Geometry check sheet. Reference: the model listing, model coordinates, mm. A direction names the side the tool comes from. Give positions to 0.01 mm unless a question says otherwise; leave off trailing zeros. Loops run counter-clockwise (first coordinate to the right, second up) from the corner with the lowest first, then second, coordinate; pieces in that order, holes last. Notation, with made-up numbers: (54.25, 50.25) -> (67.25, 50.25) arc R22 ccw to (67.25, 83.25) -> close; hole circle Ø1 at (-20, 51.5). An arc over 180 degrees is marked (long way). Answer in a Markdown table with one row per item. Add a question column.
```python
from build123d import *

# Parameters (mm, degrees)
SZKIC1_W                    = 70
SZKIC1_H                    = 100
DODANIE_WYCI_GNI_CIE1_DEPTH = 10
SZKIC2_R                    = 10
DODANIE_WYCI_GNI_CIE2_DEPTH = 30
SZKIC3_R                    = 15
DODANIE_WYCI_GNI_CIE3_DEPTH = 60
WYTNIJ_WYCI_GNI_CIE1_DEPTH  = 30


with BuildPart() as part:
    # Szkic1 → Dodanie-wyciągnięcie1 (new body)
    with BuildSketch(Plane.XY):
        Rectangle(SZKIC1_W, SZKIC1_H)
    extrude(amount=DODANIE_WYCI_GNI_CIE1_DEPTH)

    # Szkic2 → Dodanie-wyciągnięcie2 (add)
    with BuildSketch(Plane(origin=(0, 0, 0), x_dir=(-1, 0, 0), z_dir=(0, 0, -1))):
        Circle(SZKIC2_R)
    extrude(amount=DODANIE_WYCI_GNI_CIE2_DEPTH)

    # Szkic3 → Dodanie-wyciągnięcie3 (add)
    with BuildSketch(Plane(origin=(0, 0, -30), x_dir=(-1, 0, 0), z_dir=(0, 0, -1))):
        Circle(SZKIC3_R)
    extrude(amount=DODANIE_WYCI_GNI_CIE3_DEPTH)

    # Szkic4 → Wytnij-wyciągnięcie1 (cut, symmetric)
    with BuildSketch(Plane(origin=(0, 0, 0), x_dir=(0, 0, -1), z_dir=(1, 0, 0))):
        Polygon((83.125666523, 15), (44.759974282, -15), (90, -15), (90, 15), align=None)
    extrude(amount=WYTNIJ_WYCI_GNI_CIE1_DEPTH, both=True, mode=Mode.SUBTRACT)


solid = part.part
```
1. Sectioned sample at C-C (y = -13). Enter the section's corners in (x, z).
2. Gauge pin test, flat ends, axial feed: pin 1 Ø1.5 at (x, z) = (1, -35) entering from -Y; pin 2 Ø6 at (x, z) = (-19.5, -55) entering from +Y; pin 3 Ø10 at (x, y) = (-26, -1) entering from -Z; pin 4 Ø12 at (x, z) = (-16.5, -52.5) entering from +Y. Record the tip position at first contact, or that the pin passes through.
3. Sectioned sample at A-A (x = -11.5). Enter the section's corners in (y, z).
4. Access from +Z, -Z, +X, -X, +Y, -Y to the whole of each face (thin tool, end or side, straight path). Record for faces 5 (the face through (1.953, 14.872, -50.288)), 6 (the face through (0, -50, 5)).
5. Sectioned sample at B-B (x = 0). Enter the section's corners in (y, z).
6. Release check for a two-part mould opening along Z. For faces 1 (the face through (2.17, -9.76, -14.79)), 2 (the face through (0, 50, 5)), 3 (the face through (0.2, 0.2, -64.2)), 4 (the face through (-3, -10, -30)) record: released by +Z, released by -Z, zero draft, split by the parting line, or undercut.
7. Sectioned sample at D-D (z = -40). Enter the section's corners in (x, y), plus the area to 3 significant figures.
8. Material ranges on L1, parallel to Z at x = 13.5, y = -18; L2, parallel to Z at x = 8.5, y = 6; L3, parallel to X at y = 2.5, z = -40, recorded low to high. Write a range as from..to.
Response:
| question | item | result |
|---|---|---|
| 1 | outline | (-35, 0) -> (35, 0) -> (35, 10) -> (-35, 10) -> close; (-7.48, -47.32) -> (7.48, -47.32) -> (7.48, -30) -> (-7.48, -30) -> close |
| 2 | pin 1 | stops at y = -15 |
| 2 | pin 2 | passes through |
| 2 | pin 3 | stops at z = 0 |
| 2 | pin 4 | stops at y = 10.71 |
| 3 | outline | (-50, 0) -> (50, 0) -> (50, 10) -> (-50, 10) -> close; (-9.63, -51.63) -> (9.63, -76.26) -> (9.63, -30) -> (-9.63, -30) -> close |
| 4 | face 5 | -Z |
| 4 | face 6 | +Z, -Z, +X, -X, -Y |
| 5 | outline | (-50, 0) -> (-10, 0) -> (-10, -30) -> (-15, -30) -> (-15, -44.76) -> (15, -83.13) -> (15, -30) -> (10, -30) -> (10, 0) -> (50, 0) -> (50, 10) -> (-50, 10) -> close |
| 6 | face 1 | undercut |
| 6 | face 2 | zero draft |
| 6 | face 3 | released by -Z |
| 6 | face 4 | undercut |
| 7 | outline | circle Ø30 at (0, 0) |
| 7 | area | 707 mm2 |
| 8 | L1 | z = 0..10 |
| 8 | L2 | z = -71.62..-30, 0..10 |
| 8 | L3 | x = -14.79..14.79 |
